```python
from build123d import *

# Parameters (mm, degrees)
BOSS_EXTRUDE1_DEPTH = 25
CUT_EXTRUDE1_REACH  = 16
SKETCH3_W           = 14
SKETCH3_H           = 7


with BuildPart() as part:
    # Sketch2 → Boss-Extrude1 (new body, symmetric)
    with BuildSketch(Plane(origin=(0, 0, 0), x_dir=(0, 0, -1), z_dir=(1, 0, 0))):
        Polygon((0, 0), (-28, 0), (-28, 14), (-14, 14), align=None)
    extrude(amount=BOSS_EXTRUDE1_DEPTH, both=True)

    # Sketch3 → Cut-Extrude1 (cut, up to next)
    with BuildSketch(Plane(origin=(0, 14, 0), x_dir=(1, 0, 0), z_dir=(0, 1, 0)), mode=Mode.PRIVATE) as cut_extrude1_sk1:
        with Locations((3, -24.5)):
            Rectangle(SKETCH3_W, SKETCH3_H)
    cut_extrude1_tool1 = extrude(cut_extrude1_sk1.sketch, amount=-CUT_EXTRUDE1_REACH, mode=Mode.PRIVATE) & part.part
    add(cut_extrude1_tool1.solids().sort_by_distance((3, 14, 24.5))[0], mode=Mode.SUBTRACT)

    # Mirror1: part across plane


with BuildPart() as part_1:
    add(part.part)
    add(part.part.mirror(Plane(origin=(25, 14, 14), x_dir=(0, 0.707106781, 0.707106781), z_dir=(0, -0.707106781, 0.707106781))))


solid = part_1.part
```
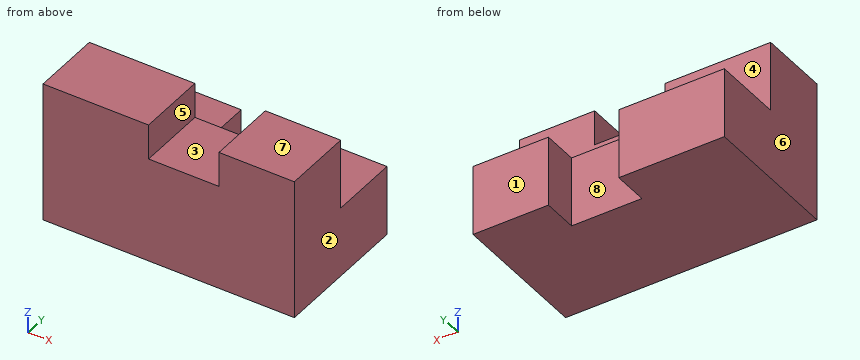
Here's how the part is built. I have some questions about the finished solid (model axes, mm). Face numbers are marked on the shaded views. A direction names the side the tool comes from. Give positions to 0.01 mm unless a question says otherwise; leave off trailing zeros. Loops run counter-clockwise (first coordinate to the right, second up) from the corner with the lowest first, then second, coordinate; pieces in that order, holes last. Notation, with made-up numbers: (-3.75, 22) -> (3.25, 22) arc R5 ccw to (3.25, 26) -> close; hole circle Ø11 at (33, 61). An arc over 180 degrees is marked (long way). Use one line per item in the form item = value. Start each with the question number.
1) Please list where these lines run through material, in increasing order: line 1 along Z through (x, y) = (8, 3.5); line 2 along X through (y, z) = (21.5, 6).
2) Thinking about a two-plate mould opening in X: for the marked faces 1, 2 and 3, which applies, +X half, -X half, draft (parallel to the pull), parting line (faces both ways), or undercut?
3) Which directions (+Z, -Z, +X, -X, +Y, -Y) give clear straight access to the entire face, cutting with the end or side of a thin tool? Please do the marked faces 4, 5, 6, 7 and 8.
4) Imagine slicing it at D-D (x = 18). Please give me the cut outline in (y, z).
5) For P1, Ø6, axis at x = -13.5, y = 18, coming from the +Z side; P2, Ø4, axis at x = 10.5, z = 21, coming from the +Y side; P3, Ø4, axis at x = 0.5, y = 9, coming from the +Z side, each with a flat end and sliding along its axis, tell me the tip position at first contact or that it passes through.
6) Imagine slicing it at A-A (y = 24.25). Please give me the cut outline in (x, z).
7) Imagine slicing it at C-C (y = 13.25). Please give me the cut outline in (x, z).
Check values:
q1.line_1 = 0 to 21
q1.line_2 = -25 to -4, 10 to 25
q2.face_1 = draft
q2.face_2 = +X half
q2.face_3 = undercut
q3.face_4 = +Z, +X, -X, +Y
q3.face_5 = +Z, +Y, -Y
q3.face_6 = +Z, -Z, -X, +Y, -Y
q3.face_7 = +Z, +X, -X, +Y, -Y
q3.face_8 = +Z, -Z, +Y
q4.outline = (0, 0) -> (28, 0) -> (28, 14) -> (14, 14) -> (14, 28) -> (0, 28) -> close
q5.P1 = 14
q5.P2 = 14
q5.P3 = 21
q6.outline = (-25, 0) -> (-4, 0) -> (-4, 14) -> (-25, 14) -> close; (10, 0) -> (25, 0) -> (25, 14) -> (10, 14) -> close
q7.outline = (-25, 0) -> (25, 0) -> (25, 28) -> (10, 28) -> (10, 21) -> (-4, 21) -> (-4, 28) -> (-25, 28) -> close
